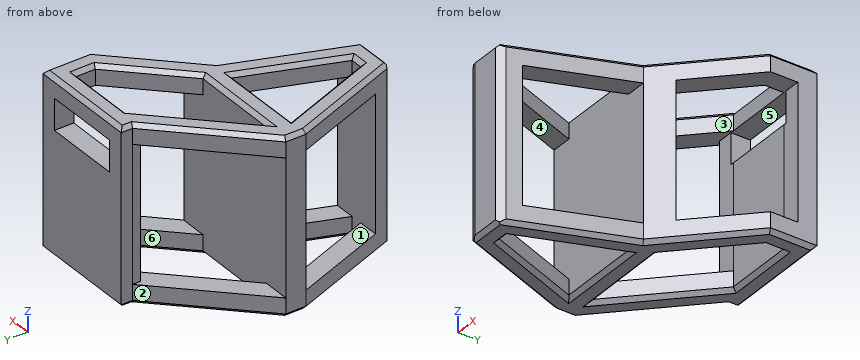
```python
from build123d import *
from OCP.BRepFilletAPI import BRepFilletAPI_MakeChamfer

# Parameters (mm, degrees)
BOSS_EXTRUDE1_DEPTH  = 5
BOSS_EXTRUDE3_DEPTH  = 5
BOSS_EXTRUDE4_DEPTH  = 26.9
SKETCH5_W            = 19.999999999999993
SKETCH5_H            = 5.000000000000007
CUT_EXTRUDE2_DEPTH   = 5.899999999999998
CUT_EXTRUDE3_DEPTH   = 2.949999999999999
BOSS_EXTRUDE5_DEPTH  = 3
BOSS_EXTRUDE6_DEPTH  = 5
BOSS_EXTRUDE7_DEPTH  = 5
BOSS_EXTRUDE8_DEPTH  = 35.00000000000001
BOSS_EXTRUDE10_DEPTH = 35.00000000000001
CHAMFER2_SIZE        = 1
CHAMFER3_SIZE        = 1
CHAMFER3_SIZE2       = 1.7100094702429673
CHAMFER3_SIZE2_2     = 1.7064334239442103


with BuildPart() as part:
    # Model → Boss-Extrude1 (new body)
    with BuildSketch(Plane.XY):
        Polygon((66.34301586992632, 59.26133691593834), (66.3616632211768, 66.2613120784865), (38.072757817888686, 66.41203172728402), (38.064905748927345, 63.464466308167324), (14.948145869822214, 40.47054145556226), (14.934248363068548, 35.253596657867014), (26.03420495541168, 5.596834863804027), (36.03420495541168, 5.596834863804027), (47.134161547754815, 35.167818769025025), (66.32969633331885, 54.261354656975335), align=None)
        Polygon((20.278317449078216, 35.23936050258937), (41.79885052391343, 35.18203159355395), (32.57039139015228, 10.596834863804013), (29.501541711242254, 10.596834863804041), align=None, mode=Mode.SUBTRACT)
        Polygon((43.06467722097951, 61.38536445785425), (61.3483968604827, 61.28795115170147), (61.3352312070632, 56.345734656870185), (45.076420621075016, 40.17331816069535), (21.96849830021793, 40.4012838462993), align=None, mode=Mode.SUBTRACT)
    extrude(amount=BOSS_EXTRUDE1_DEPTH)

    # Sketch3 → Boss-Extrude3 (add)
    with BuildSketch(Plane.XY.offset(5)):
        Polygon((66.36166322117678, 66.2613120784865), (38.072757817888686, 66.41203172728402), (38.064905748927345, 63.464466308167324), (38.064905748927345, 61.38536445785425), (43.06467722097951, 61.38536445785425), (61.3483968604827, 61.28795115170147), (66.34841460158263, 61.28795115170147), align=None)
    extrude(amount=BOSS_EXTRUDE3_DEPTH)

    # Sketch4 → Boss-Extrude4 (add)
    with BuildSketch(Plane.XY.offset(10)):
        Polygon((66.34841460158263, 61.28795115170147), (66.36166322117678, 66.2613120784865), (38.072757817888686, 66.41203172728402), (38.064905748927345, 63.464466308167324), (38.064905748927345, 61.38536445785425), (43.06467722097951, 61.38536445785425), (61.3483968604827, 61.28795115170147), align=None)
    extrude(amount=BOSS_EXTRUDE4_DEPTH)

    # Sketch5 → Cut-Extrude2 (cut)
    with BuildSketch(Plane(origin=(0.3282664498542539, 61.613058556670126, 0), x_dir=(0.999985807195565, -0.005327795738801082, 0), z_dir=(-0.005327795738801082, -0.999985807195565, 0))):
        with Locations((51.87900689947605, 34.400000000000006)):
            Rectangle(SKETCH5_W, SKETCH5_H)
    extrude(amount=-CUT_EXTRUDE2_DEPTH, mode=Mode.SUBTRACT)

    # Sketch7 → Cut-Extrude3 (cut, symmetric)
    with BuildSketch(Plane(origin=(0.32826644985427067, 61.61305855667014, 0), x_dir=(0.999985807195565, -0.005327795738801352, 0), z_dir=(0.005327795738801352, 0.999985807195565, 0))):
        Polygon((42.73701732925542, -31.9), (41.87900689947603, -31.9), (41.87900689947603, -36.900000000000006), (42.73701732945169, -36.900000000000006), align=None)
    extrude(amount=CUT_EXTRUDE3_DEPTH, both=True, mode=Mode.SUBTRACT)

    # Sketch8 → Boss-Extrude5 (add)
    with BuildSketch(Plane.XY.offset(36.900000000000006)):
        Polygon((38.064905748927345, 61.38536445785425), (42.20665461345415, 61.385364457854244), (42.23331794746946, 66.38986479814373), (38.072757817888686, 66.41203172728402), (38.064905748927345, 63.464466308167324), align=None)
        Polygon((66.36166322117678, 66.2613120784865), (62.23303409138075, 66.28330888336767), (62.20641946800804, 61.28795115170146), (66.34841460158263, 61.28795115170147), align=None)
    extrude(amount=BOSS_EXTRUDE5_DEPTH)

    # Sketch9 → Boss-Extrude6 (add)
    with BuildSketch(Plane.XY.offset(39.900000000000006)):
        Polygon((62.233034091380745, 66.28330888336767), (42.23331794746946, 66.38986479814372), (42.20665461345415, 61.38536445785425), (43.064677220980606, 61.38536445785425), (61.3483968604827, 61.28795115170147), (62.20641946800805, 61.28795115170147), align=None)
        Polygon((42.23331794746946, 66.38986479814373), (38.072757817888686, 66.41203172728402), (38.064905748927345, 63.464466308167324), (38.064905748927345, 61.38536445785425), (42.20665461345415, 61.385364457854244), align=None)
        Polygon((62.20641946800804, 61.28795115170146), (66.34841460158263, 61.28795115170147), (66.36166322117678, 66.2613120784865), (62.23303409138075, 66.28330888336767), align=None)
    extrude(amount=BOSS_EXTRUDE6_DEPTH)

    # Sketch10 → Boss-Extrude7 (add)
    with BuildSketch(Plane.XY.offset(44.900000000000006)):
        Polygon((66.34841460158262, 61.28795115170147), (61.3483968604827, 61.28795115170147), (61.3352312070632, 56.34573465687018), (45.076420621075016, 40.17331816069535), (21.968498300217927, 40.4012838462993), (43.06467722097951, 61.38536445785425), (38.064905748927345, 61.38536445785425), (38.064905748927345, 63.464466308167324), (14.948145869822214, 40.470541455562255), (14.934248363068548, 35.25359665786701), (26.03420495541168, 5.596834863804027), (36.03420495541168, 5.596834863804027), (47.134161547754815, 35.16781876902502), (66.32969633331884, 54.261354656975335), align=None)
        Polygon((29.50154171124225, 10.596834863804041), (32.57039139015229, 10.596834863804013), (41.79885052391343, 35.18203159355396), (20.278317449078216, 35.23936050258938), align=None, mode=Mode.SUBTRACT)
    extrude(amount=-BOSS_EXTRUDE7_DEPTH)

    # Sketch11 → Boss-Extrude8 (add)
    with BuildSketch(Plane.XY.offset(5)):
        Polygon((24.162800944848858, 10.596834863804041), (26.03420495541168, 5.596834863804027), (36.03420495541168, 5.596834863804027), (37.91103743212602, 10.596834863804041), align=None)
    extrude(amount=BOSS_EXTRUDE8_DEPTH)

    # Sketch12 → Boss-Extrude10 (add)
    with BuildSketch(Plane.XY.offset(5)):
        Polygon((52.096773051470755, 40.1040605514324), (14.948145869822214, 40.470541455562255), (14.934248363068548, 35.25359665786701), (47.134161547754815, 35.16781876902502), align=None)
    extrude(amount=BOSS_EXTRUDE10_DEPTH)

    # Chamfer2
    chamfer2_edges = [part.edges().sort_by_distance(p)[0] for p in [
        (52.217210519532735, 66.33667190288526, 44.900000000000006),
        (38.068831783408015, 64.93824901772567, 44.900000000000006),
        (52.206537040731654, 61.33665780477786, 44.900000000000006),
        (66.34567977724781, 60.26133336773091, 44.900000000000006),
        (20.484226659240115, 20.42521576083552, 0),
        (14.94119711644538, 37.86206905671464, 0),
        (26.50652580937478, 51.9675038818648, 0),
        (38.068831783408015, 64.93824901772567, 0),
        (61.34181403377295, 58.81684290428582, 44.900000000000006),
        (53.20582591406911, 48.25952640878276, 44.900000000000006),
        (33.52245946064647, 40.287301003497326, 44.900000000000006),
        (32.51658776059872, 50.89332415207677, 44.900000000000006),
        (52.21721051953274, 66.33667190288526, 0),
        (26.50652580937478, 51.967503881864786, 44.900000000000006),
        (14.94119711644538, 37.86206905671463, 44.900000000000006),
        (20.484226659240115, 20.425215760835517, 44.900000000000006),
        (31.03420495541168, 5.596834863804027, 44.900000000000006),
        (41.58418325158325, 20.382326816414523, 44.900000000000006),
        (56.731928940536825, 44.71458671300017, 44.900000000000006),
        (24.889929580160235, 22.91809768319671, 44.900000000000006),
        (31.038583986495823, 35.21069604807167, 44.900000000000006),
        (37.18462095703286, 22.889433228678985, 44.900000000000006),
        (31.035966550697268, 10.596834863804027, 44.900000000000006),
        (66.34567977724782, 60.26133336773091, 0),
        (56.73192894053683, 44.71458671300018, 0),
        (41.58418325158325, 20.382326816414526, 0),
        (31.03420495541168, 5.596834863804027, 0),
        (53.20582591406911, 48.25952640878277, 0),
        (61.34181403377295, 58.81684290428583, 0),
        (52.20653704073111, 61.33665780477786, 0),
        (32.516587760598725, 50.89332415207678, 0),
        (33.52245946064647, 40.287301003497326, 0),
        (37.184620957032855, 22.889433228678982, 0),
        (31.038583986495823, 35.21069604807166, 0),
        (24.889929580160235, 22.918097683196706, 0),
        (31.035966550697268, 10.596834863804027, 0),
    ]]
    chamfer(chamfer2_edges, length=CHAMFER2_SIZE)

    # Chamfer3: one chamfer whose edges measure the first distance from different faces: ONE call of the kernel's chamfer builder (chamfer() names one face for all edges)
    chamfer3_edges_1 = [part.edges().sort_by_distance(p)[0] for p in [
        (36.03420495541168, 5.596834863804027, 22.450000000000003),
    ]]
    chamfer3_side_1 = [part.faces().sort_by_distance(p)[0] for p in [
        (31.03420495541168, 5.596834863804027, 22.450000000000003),
    ]]
    chamfer3_edges_2 = [part.edges().sort_by_distance(p)[0] for p in [
        (26.03420495541168, 5.596834863804027, 22.450000000000003),
    ]]
    chamfer3_side_2 = [part.faces().sort_by_distance(p)[0] for p in [
        (15.121156427701985, 34.75421741218178, 3),
    ]]
    chamfer3 = BRepFilletAPI_MakeChamfer(part.part.solid().wrapped)
    for e in chamfer3_edges_1:
        chamfer3.Add(CHAMFER3_SIZE, CHAMFER3_SIZE2, e.wrapped, chamfer3_side_1[0].wrapped)  # the first distance lies on this face
    for e in chamfer3_edges_2:
        chamfer3.Add(CHAMFER3_SIZE, CHAMFER3_SIZE2_2, e.wrapped, chamfer3_side_2[0].wrapped)  # the first distance lies on this face
    add(Compound.cast(chamfer3.Shape()), mode=Mode.REPLACE)


solid = part.part
```
Verification items for the finished model (mm, model axes). Face numbers are marked on the shaded views. A direction names the side the tool comes from. Coordinates: 2 decimals unless noted, no trailing zeros. Write each loop counter-clockwise with the first axis right and the second up, starting at its lowest first coordinate (ties: lowest second). Pieces come first, ordered by that corner, then holes. Notation, with made-up numbers: M 41,68 L 46,68 A25 cw 46,85 Z; hole C -38.75,39.25 d6. An arc over 180 degrees is marked long. One line per item, written item: value.
Item 1: Section check B-B, the plane z = 41.5. Record the boundary of the cut face in (x, y), plus the area to 3 significant figures.
Check sheet entries:
outline: M 14.93,35.25 L 25.68,6.53 L 27.74,5.6 L 35.03,5.6 L 36.64,7.2 L 47.13,35.17 L 66.33,54.26 L 66.36,66.26 L 38.07,66.41 L 38.06,63.46 L 14.95,40.47 Z; hole M 20.28,35.24 L 29.5,10.6 L 32.57,10.6 L 41.8,35.18 Z; hole M 21.97,40.4 L 45.08,40.17 L 61.34,56.35 L 61.35,61.29 L 43.06,61.39 Z
area: 927 mm^2
Item 2: Mould release check, pull along X, two halves, no side actions. Record for the marked faces 1, 2 and 3: pulls with the +X half, pulls with the -X half, needs draft (parallel to the pull), parting line crosses it, or undercut.
Check sheet entries:
face 1: needs draft
face 2: pulls with the -X half
face 3: undercut
Item 3: Section check A-A, the plane z = 30. Record the boundary of the cut face in (x, y).
Check sheet entries:
outline: M 14.93,35.25 L 47.13,35.17 L 52.1,40.1 L 14.95,40.47 Z; M 24.16,10.6 L 25.68,6.53 L 27.74,5.6 L 35.03,5.6 L 36.64,7.2 L 37.91,10.6 Z; M 38.06,61.39 L 43.06,61.39 L 61.35,61.29 L 66.35,61.29 L 66.36,66.26 L 38.07,66.41 L 38.06,63.46 Z
Item 4: Section check D-D, the plane x = 57.5. Record the boundary of the cut face in (y, z), plus the area to 3 significant figures.
Check sheet entries:
outline: M 45.48,1 L 46.89,0 L 51.12,0 L 52.53,1 L 52.53,5 L 45.48,5 Z; M 45.48,39.9 L 52.53,39.9 L 52.53,43.9 L 51.12,44.9 L 46.89,44.9 L 45.48,43.9 Z; M 61.31,1 L 62.31,0 L 65.31,0 L 66.31,1 L 66.31,31.9 L 61.31,31.9 Z; M 61.31,39.9 L 66.31,39.9 L 66.31,43.9 L 65.31,44.9 L 62.31,44.9 L 61.31,43.9 Z
area: 250 mm^2
Item 5: Gauge pin test, flat ends, axial feed: pin 1 Ø16 at (x, y) = (20.5, 18.5) entering from -Z; pin 2 Ø8 at (y, z) = (58, 34) entering from +X; pin 3 Ø4.5 at (x, y) = (36.5, 28) entering from -Z; pin 4 Ø2.5 at (x, z) = (41.5, 24) entering from -Y. Record the tip position at first contact, or that the pin passes through.
Check sheet entries:
pin 1: stops at z = 0
pin 2: stops at x = 66.35
pin 3: passes through
pin 4: stops at y = 35.18
Item 6: Scan lines: line 1 along Z through (x, y) = (28, 49.5); line 2 along Y through (x, z) = (49, 18); line 3 along X through (y, z) = (52.5, 4). Record each from-to range of solid material in increasing order.
Check sheet entries:
line 1: z = 0 to 5, 39.9 to 44.9
line 2: y = 37.02 to 40.13, 61.35 to 66.35
line 3: x = 27.04 to 34.13, 57.47 to 64.56
Item 7: Section check C-C, the plane y = 45.5. Record the boundary of the cut face in (x, z), plus the area to 3 significant figures.
Check sheet entries:
outline: M 20,1 L 21.42,0 L 25.68,0 L 27.09,1 L 27.09,5 L 20,5 Z; M 20,39.9 L 27.09,39.9 L 27.09,43.9 L 25.68,44.9 L 21.42,44.9 L 20,43.9 Z; M 50.43,1 L 51.85,0 L 56.1,0 L 57.52,1 L 57.52,5 L 50.43,5 Z; M 50.43,39.9 L 57.52,39.9 L 57.52,43.9 L 56.1,44.9 L 51.85,44.9 L 50.43,43.9 Z
area: 136 mm^2
Item 8: Access from +Z, -Z, +X, -X, +Y, -Y to the whole of each face (thin tool, end or side, straight path). Record for the marked faces 4, 5 and 6.
Check sheet entries:
face 4: +X, -X
face 5: none
face 6: +Z, -Z
